Can you work these out from the model? Positions are in its coordinate system, mm. A direction names the side the tool comes from. Give positions to 0.01 mm unless a question says otherwise; leave off trailing zeros. Write each loop counter-clockwise with the first axis right and the second up, starting at its lowest first coordinate (ties: lowest second). Pieces come first, ordered by that corner, then holes. Notation, with made-up numbers: (-31, 54) -> (-22, 54) arc R17 cw to (-22, 81) -> close; hole circle Ø8 at (39.5, -11.75). An arc over 180 degrees is marked (long way). Answer as CSV lines item,"result". Start each with the question number.
1. If we section it at A-A on x = 3.05: Write out the boundary of the cut face in (y, z) (3 decimals).
2. On a 3-axis mill with a long thin cutter (end or side, diameter ignored), from which of +Z, -Z, +X, -X, +Y, -Y can I reach the whole of each face in a straight line? I mean faces 5 (the face through (3, 4.5, -230)), 6 (the face through (3, 10, 0)). Say none if no direction works.
3. If we section it at B-B on z = -15: Write out the boundary of the cut face in (x, y) (3 decimals).
4. I need wall thicknesses on line 1 (Z direction, x = 4.7, y = 6) (3 decimals); line 2 (Y direction, x = 2.2, z = -237.46); line 3 (Z direction, x = 4.85, y = 6.5). Which ranges of each line are inside material? Lowest first, please. Write a range as [from, to].
5. If we mould it in two halves opening along Y, with no side actions, what happens to faces 1 (the face through (3, 0, -142)), 2 (the face through (3, 10, -280)), 3 (the face through (3, 20, -138)), 4 (the face through (2.96, 5.31, -261.9))? For each: pulls with the +Y half, pulls with the -Y half, needs draft (parallel to the pull), parting line crosses it, or undercut.
Autodesk Inventor part; units mm, degrees
ref_plane "YZ Plane" through (0, 0, 0) normal (1, 0, 0) x (0, 1, 0)
ref_plane "XZ Plane" through (0, 0, 0) normal (0, 1, 0) x (-1, 0, 0)
ref_plane "XY Plane" through (0, 0, 0) normal (0, 0, 1) x (1, 0, 0)
sketch "Boceto1" plane through (0, 0, 0) normal (1, 0, 0) x (0, 1, 0)
  line L0 (0, 0) -> (20, 0)
  line L1 (20, 0) -> (20, -280)
  line L2 (20, -280) -> (0, -280)
  line L3 (0, -280) -> (0, 0)
  circle A0 centre (6, -15) radius 3.175
  circle A1 centre (6, -265) radius 3.175
  dimension "d0" = 20
  dimension "d1" = 280
  dimension "d2" = 6.35
  dimension "d8" = 6
  dimension "d9" = 250
  dimension "d10" = 15
extrude "Extrusión1" add sketch "Boceto1" along normal blind 6
sketch "Boceto2" plane through (6, 0, 0) normal (1, 0, 0) x (0, 0, -1)
  line L0 (220, 17.5) -> (240, 17.5)
  line L1 (240, 17.5) -> (240, 2.5)
  line L2 (240, 2.5) -> (220, 2.5)
  line L3 (220, 2.5) -> (220, 17.5)
  line L4 (280, 0) -> (280, 20)
  line L5 (240, 2.5) -> (220, 2.5)
  line L6 (220, 2.5) -> (220, 4.5)
  line L7 (220, 4.5) -> (240, 4.5)
  line L8 (240, 4.5) -> (240, 2.5)
  circle A0 centre (222.54, 14.96) radius 1.5
  line L9 (230, 17.5) -> (230, 4.5)
  circle A1 centre (237.46, 14.96) radius 1.5
  point P0 (0, 0)
  point P1 (240, 10)
  point P2 (280, 10)
  dimension "d11" = 20
  dimension "d12" = 15
  dimension "d13" = 40
  dimension "d14" = 2
  dimension "d15" = 3
  dimension "d16" = 2.54
  dimension "d17" = 2.54
extrude "Extrusión2" cut sketch "Boceto2" against normal through all contours L7 L1 L2 L3 | A0 | A1
properties part number "Riel_Lateral_MDF"
Computed values:
1,outline,"(0, -280) -> (20, -280) -> (20, 0) -> (0, 0) -> close; hole (2.5, -240) -> (4.5, -240) -> (4.5, -220) -> (2.5, -220) -> close; hole circle Ø6.35 at (6, -265); hole circle Ø6.35 at (6, -15); hole circle Ø3 at (14.96, -237.46); hole circle Ø3 at (14.96, -222.54)"
2,face 5,"+X, -X"
2,face 6,"+Z, +X, -X, +Y, -Y"
3,outline,"(0, 0) -> (6, 0) -> (6, 2.825) -> (0, 2.825) -> close; (0, 9.175) -> (6, 9.175) -> (6, 20) -> (0, 20) -> close"
4,line 1,"z = [-280, -268.175], [-261.825, -18.175], [-11.825, 0]"
4,line 2,"y = [0, 2.5], [4.5, 13.46], [16.46, 20]"
4,line 3,"z = [-280, -268.14], [-261.86, -18.14], [-11.86, 0]"
5,face 1,"pulls with the -Y half"
5,face 2,"needs draft"
5,face 3,"pulls with the +Y half"
5,face 4,"undercut"
